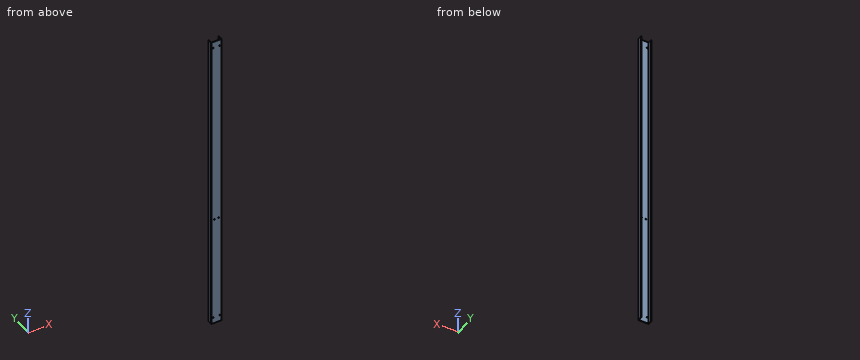
```python
from build123d import *

# Parameters (mm, degrees)
SM_BASE_FLANGE_1_DEPTH    = 950
HOLE_WIZARD_6_0_6_1_D     = 6
HOLE_WIZARD_6_0_6_1_DEPTH = 15
HOLE_WIZARD_6_0_6_1_TIP   = 1.802581857
HOLE_WIZARD_6_5_6_5_1_D   = 6.5


# Sheet-metal steps are written as plain solids
with BuildPart() as part:
    # Sketch 1 → 基体-法兰1 (new, symmetric)
    with BuildSketch(Plane.XY):
        with BuildLine():
            Line((-30, 25), (-30, 0.7366))
            ThreePointArc((-30, 0.7366), (-29.784254855, 0.215745145), (-29.2634, 0))
            Line((-29.2634, 0), (29.2634, 0))
            ThreePointArc((29.2634, 0), (29.784254855, 0.215745145), (30, 0.7366))
            Line((30, 0.7366), (30, 25))
            Line((30, 25), (32, 25))
            Line((32, 25), (32, 0.7366))
            ThreePointArc((32, 0.7366), (31.198468417, -1.198468417), (29.2634, -2))
            Line((29.2634, -2), (-29.2634, -2))
            ThreePointArc((-29.2634, -2), (-31.198468417, -1.198468417), (-32, 0.7366))
            Line((-32, 0.7366), (-32, 25))
            Line((-32, 25), (-30, 25))
        make_face()
    extrude(amount=SM_BASE_FLANGE_1_DEPTH, both=True)

    # Ø6.0 (6) 直径孔1
    with Locations(Plane(origin=(-20, 0, -910), x_dir=(1, 0, 0), z_dir=(0, 1, 0))):
        with Locations((0, 0), (40, 0), (0, -1820), (40, -1820)):
            Hole(HOLE_WIZARD_6_0_6_1_D / 2, depth=HOLE_WIZARD_6_0_6_1_DEPTH)
            with Locations((0, 0, -(HOLE_WIZARD_6_0_6_1_DEPTH + HOLE_WIZARD_6_0_6_1_TIP / 2))):  # 118° drill point
                Cone(0, HOLE_WIZARD_6_0_6_1_D / 2, HOLE_WIZARD_6_0_6_1_TIP, mode=Mode.SUBTRACT)

    # Ø6.5 (6.5) 直径孔1 (through all)
    with Locations(Plane(origin=(-12.5, 0, -250), x_dir=(1, 0, 0), z_dir=(0, 1, 0))):
        with Locations((0, 0), (25, 0)):
            Hole(HOLE_WIZARD_6_5_6_5_1_D / 2)


solid = part.part
```
Work out the finished part from the listing and answer in its coordinate system (mm). Round coordinates to 2 decimals unless told otherwise and drop trailing zeros. Write each loop counter-clockwise with the first axis right and the second up, starting at its lowest first coordinate (ties: lowest second). Pieces come first, ordered by that corner, then holes. Notation, with made-up numbers: (73, -23.5) - (104, -23.5) arc R13 ccw to (104, -5.5) - close; hole circle Ø5 at (2.25, 73). An arc over 180 degrees is marked (long way). Return JSON: item names as keys, results as strings. Group by question number.
Q1. The part is cut by section A-A on y = 15. Write down the section's boundary in (x, z).
Q2. Find the intervals of material crossed by L1, parallel to X at y = -0.35, z = 910; L2, parallel to Z at x = 20, y = -0.85; L3, parallel to Z at x = -12.5, y = -1.2, in increasing order.
Q3. The part is cut by section B-B on z = -556. Write down the section's boundary in (x, y).
Q4. This flat-tipped pin is pushed along its axis until it touches: pin 1 Ø4 at (x, z) = (-10, -508.5) entering from +Y. Where does it stop, or does it pass through?
Solved:
{
 "1": {"outline": "(-32, -950) - (-30, -950) - (-30, 950) - (-32, 950) - close; (30, -950) - (32, -950) - (32, 950) - (30, 950) - close"},
 "2": {"L1": "-31.78 to -23, -17 to 17, 23 to 31.78", "L2": "-950 to -913, -907 to 907, 913 to 950", "L3": "-950 to -253.25, -246.75 to 950"},
 "3": {"outline": "(-32, 0.74) arc R2.74 ccw to (-29.26, -2) - (29.26, -2) arc R2.74 ccw to (32, 0.74) - (32, 25) - (30, 25) - (30, 0.74) arc R0.74 cw to (29.26, 0) - (-29.26, 0) arc R0.74 cw to (-30, 0.74) - (-30, 25) - (-32, 25) - close"},
 "4": {"pin 1": "y = 0"}
}
